from build123d import *

# Parameters (mm, degrees)
BOX014_W          = 15
BOX014_H          = 1.6
BOX014_DEPTH      = 10.5
CYLINDER024_R     = 2.9
CYLINDER024_DEPTH = 10.5
CYLINDER023_R     = 4.5
CYLINDER023_DEPTH = 7
CYLINDER022_R     = 14.7
CYLINDER022_DEPTH = 20.5
CYLINDER021_R     = 16.3
CYLINDER021_DEPTH = 20.5
CHAMFER010_SIZE   = 1.6
CHAMFER011_SIZE   = 1.6
CHAMFER012_SIZE   = 1.6


with BuildPart() as obj1:
    # Box014 → Box014 (new body)
    with BuildSketch(Plane(origin=(123, 18.3, 1.6), x_dir=(1, 0, 0), z_dir=(0, 0, 1))):
        with Locations((7.5, 0.8)):
            Rectangle(BOX014_W, BOX014_H)
    extrude(amount=BOX014_DEPTH)


with BuildPart() as zylinder024:
    # Cylinder024 → Cylinder024 (new body)
    with BuildSketch(Plane(origin=(130, 19.1, 1.6), x_dir=(1, 0, 0), z_dir=(0, 0, 1))):
        Circle(CYLINDER024_R)
    extrude(amount=CYLINDER024_DEPTH)


with BuildPart() as cut016:
    # Cylinder023 → Cylinder023 (new body)
    with BuildSketch(Plane(origin=(130, 19.1, 0), x_dir=(1, 0, 0), z_dir=(0, 0, 1))):
        Circle(CYLINDER023_R)
    extrude(amount=CYLINDER023_DEPTH)

    # Cut016: cut Zylinder024
    add(zylinder024.part, mode=Mode.SUBTRACT)


with BuildPart() as zylinder022:
    # Cylinder022 → Cylinder022 (new body)
    with BuildSketch(Plane(origin=(130, 19.1, 1.6), x_dir=(1, 0, 0), z_dir=(0, 0, 1))):
        Circle(CYLINDER022_R)
    extrude(amount=CYLINDER022_DEPTH)


with BuildPart() as knob_big:
    # Cylinder021 → Cylinder021 (new body)
    with BuildSketch(Plane(origin=(130, 19.1, 0), x_dir=(1, 0, 0), z_dir=(0, 0, 1))):
        Circle(CYLINDER021_R)
    extrude(amount=CYLINDER021_DEPTH)

    # Cut015: cut Zylinder022
    add(zylinder022.part, mode=Mode.SUBTRACT)

    # Chamfer010
    chamfer010_edges = [knob_big.edges().sort_by_distance(p)[0] for p in [
        (115.3, 19.1, 1.6),
    ]]
    chamfer(chamfer010_edges, length=CHAMFER010_SIZE)

    # Chamfer011
    chamfer011_edges = [knob_big.edges().sort_by_distance(p)[0] for p in [
        (113.7, 19.1, 0),
    ]]
    chamfer(chamfer011_edges, length=CHAMFER011_SIZE)

    # Fusion014: union Cut016
    add(cut016.part)

    # Chamfer012
    chamfer012_edges = [knob_big.edges().sort_by_distance(p)[0] for p in [
        (125.5, 19.1, 1.6),
    ]]
    chamfer(chamfer012_edges, length=CHAMFER012_SIZE)

    # Cut017: cut obj1
    add(obj1.part, mode=Mode.SUBTRACT)


with BuildPart() as knob_big_1:
    # Cut017 placement: moved
    add(knob_big.part.moved(Location((40, 0, 0))))


solid = knob_big_1.part
The model under review builds one solid part; all positions refer to its coordinate system, in mm. A direction names the side the tool comes from. Give positions to 0.01 mm unless a question says otherwise; leave off trailing zeros. Write each loop counter-clockwise with the first axis right and the second up, starting at its lowest first coordinate (ties: lowest second). Pieces come first, ordered by that corner, then holes. Notation, with made-up numbers: M -32.5,35.25 L 16.5,35.25 A17 cw 16.5,55.25 Z; hole C -33.75,14 d3. An arc over 180 degrees is marked long. One line per question, with ' | ' between items. Start each with the question number.
Item 1: Wall thickness on line 1 (Y direction, x = 170, z = 14); line 2 (Z direction, x = 171, y = 11.5); line 3 (X direction, y = 23, z = 6) (3 decimals): over which ranges is each line inside the solid? List them lowest first. Write a range as from..to.
Item 2: For faces 5 (the flat face through (168, 34, 20.5)), 6 (the flat face through (166, 18.3, 4)), list the 3-axis set-ups (+Z, -Z, +X, -X, +Y, -Y) from which the entire face can be reached by the end or side of a thin tool; tool diameter is ignored.
Item 3: For pin 1 (1.1 mm diameter, centred on x = 169, y = 16, fed in from +Z); pin 2 (1.6 mm diameter, centred on x = 165, z = 4.5, fed in from -Y); pin 3 (8 mm diameter, centred on x = 179, z = 5, fed in from +Y), all flat-tipped, find the tip position at first contact; note any pin that passes through.
Item 4: We need section B-B on y = 19.1. Write out the cut boundary in (x, z), plus the area to 3 significant figures.
Item 5: Draft analysis for pull direction Y (two halves, no side actions). For faces 1 (the cylindrical face through (185.547, 23.996, 10.918)), 2 (the cylindrical face through (155.314, 19.746, 11.729)), 3 (the flat face through (174, 18.3, 4)), 4 (the flat face through (170, 19, 0)), state which applies: released by +Y, released by -Y, zero draft, split by the parting line, or undercut.
Item 6: We need section A-A on x = 170. Write out the cut boundary in (y, z), plus the area to 3 significant figures.
Item 7: We need section C-C on z = 11.5. Write out the cut boundary in (x, y).
Results found:
1) line 1: y = 2.8..4.4, 33.8..35.4 | line 2: z = 0..1.6 | line 3: x = 154.173..155.827, 167.755..172.245, 184.173..185.827
2) face 5: +Z, +X, -X, +Y, -Y | face 6: +Z
3) pin 1: stops at z = 7 | pin 2: stops at y = 3.35 | pin 3: stops at y = 34.61
4) outline: M 153.7,1.6 L 155.3,0 L 184.7,0 L 186.3,1.6 L 186.3,20.5 L 184.7,20.5 L 184.7,3.2 L 183.1,1.6 L 156.9,1.6 L 155.3,3.2 L 155.3,20.5 L 153.7,20.5 Z | area: 113 mm2
5) face 1: split by the parting line | face 2: undercut | face 3: undercut | face 4: zero draft
6) outline: M 2.8,1.6 L 4.4,0 L 33.8,0 L 35.4,1.6 L 35.4,20.5 L 33.8,20.5 L 33.8,3.2 L 32.2,1.6 L 25.2,1.6 L 23.6,3.2 L 23.6,7 L 22,7 L 22,1.6 L 16.2,1.6 L 16.2,7 L 14.6,7 L 14.6,3.2 L 13,1.6 L 6,1.6 L 4.4,3.2 L 4.4,20.5 L 2.8,20.5 Z | area: 132 mm2
7) outline: C 170,19.1 d32.6; hole C 170,19.1 d29.4
